Read the model definition and answer for the solid it produces. Units are mm, in the model's axes. Face numbers are marked on the shaded views. A direction names the side the tool comes from. Coordinates: 2 decimals unless noted, no trailing zeros. Order: outer loops, then holes, each group sorted by start corner. A loop starts at its lowest first (then second) coordinate and runs counter-clockwise, first axis right, second up. Notation, with made-up numbers: (42.25, -16) - (76.25, -16) arc R9 cw to (76.25, -11) - close; hole circle Ø4 at (24.5, -40). An arc over 180 degrees is marked (long way). Write item = value, one per line.
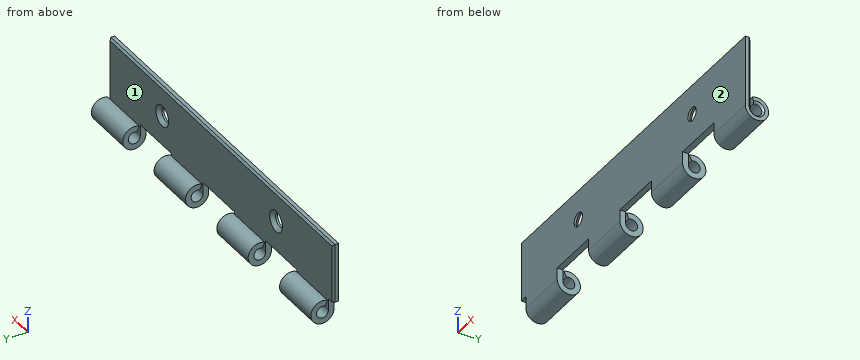
from build123d import *

# Parameters (mm, degrees)
SKETCH1_W          = 100
SKETCH1_H          = 22.1615
BASE_FLANGE1_DEPTH = 1.524
HEM1_START         = -50
HEM1_DEPTH         = 100
HEM1_2_DEPTH       = 100
CUT_EXTRUDE1_START = -52.42823759
SKETCH8_W          = 14
SKETCH8_H          = 6.223
CUT_EXTRUDE1_DEPTH = 94.856475179
LPATTERN1_COUNT    = 11
LPATTERN1_PITCH    = 28
CHAMFER1_SIZE      = 0.5
SKETCH9_R          = 1.8288
CUT_EXTRUDE2_DEPTH = 10
LPATTERN2_COUNT    = 6
LPATTERN2_PITCH    = 50.8
CHAMFER2_SIZE      = 1


# Read off the part's stored shape, not the designer's step: Hem1
# Sheet-metal steps are written as plain solids
with BuildPart() as part:
    # Sketch1 → Base-Flange1 (new body)
    with BuildSketch(Plane(origin=(0, 0, 0), x_dir=(1, 0, 0), z_dir=(0, 1, 0))):
        Rectangle(SKETCH1_W, SKETCH1_H)
    extrude(amount=-BASE_FLANGE1_DEPTH)

    # Hem1 outline → Hem1 (cut)
    with BuildSketch(Plane.YZ.offset(HEM1_START)):
        with BuildLine():
            Line((0, -11.08075), (0, -10.645306054))
            ThreePointArc((0, -10.645306054), (-1.116287945, -9.509043168), (-1.524, -7.96925))
            Line((-1.524, -7.96925), (-1.524, -11.08075))
            Line((-1.524, -11.08075), (0, -11.08075))
        make_face()
    extrude(amount=HEM1_DEPTH, mode=Mode.SUBTRACT)

    # Hem1 2 outline → Hem1 2 (add)
    with BuildSketch(Plane.YZ.offset(HEM1_START)):
        with BuildLine():
            Line((0.272523279, -5.149273321), (0.916593509, -6.530486388))
            ThreePointArc((0.916593509, -6.530486388), (2.92638392, -8.822213128), (0, -7.96925))
            Line((0, -7.96925), (0, -10.645306054))
            ThreePointArc((0, -10.645306054), (4.69518189, -8.123345818), (0.272523279, -5.149273321))
        make_face()
    extrude(amount=HEM1_2_DEPTH)

    # Sketch8 → Cut-Extrude1 (cut)
    with BuildSketch(Plane(origin=(0, 0, 0), x_dir=(1, 0, 0), z_dir=(0, 1, 0)).offset(CUT_EXTRUDE1_START)):
        with Locations((29, 7.96925)):
            Rectangle(SKETCH8_W, SKETCH8_H)
    cut_extrude1 = extrude(amount=CUT_EXTRUDE1_DEPTH, mode=Mode.SUBTRACT)

    # LPattern1: Cut-Extrude1 ×11
    with Locations(*[(-i * LPATTERN1_PITCH, 0, 0) for i in range(1, LPATTERN1_COUNT)]):
        add(cut_extrude1, mode=Mode.SUBTRACT)

    # Chamfer1
    chamfer1_edges = [part.edges().sort_by_distance(p)[0] for p in [
        (-50, 0, 3.1115),
        (50, 2.92638392, -8.822213128),
        (0, 0, 11.08075),
        (50, 0, 1.55575),
    ]]
    chamfer(chamfer1_edges, length=CHAMFER1_SIZE)

    # Sketch9 → Cut-Extrude2 (cut)
    with BuildSketch(Plane(origin=(0, 0, 0), x_dir=(1, 0, 0), z_dir=(0, 1, 0))):
        with Locations(Location((-24.6, -3.14325, 0), (0, 0, 270))):
            Circle(SKETCH9_R)
    cut_extrude2 = extrude(amount=-CUT_EXTRUDE2_DEPTH, mode=Mode.SUBTRACT)

    # LPattern2: Cut-Extrude2 ×6
    with Locations(*[(i * LPATTERN2_PITCH, 0, 0) for i in range(1, LPATTERN2_COUNT)]):
        add(cut_extrude2, mode=Mode.SUBTRACT)

    # Chamfer2
    chamfer2_edges = [part.edges().sort_by_distance(p)[0] for p in [
        (-24.6, 0, 1.31445),
        (26.2, 0, 1.31445),
    ]]
    chamfer(chamfer2_edges, length=CHAMFER2_SIZE)


solid = part.part
1) For the marked faces 1 and 2, determine the directions among +Z, -Z, +X, -X, +Y, -Y from which every point of the face is accessible in a straight line to the end or side of a thin tool.
Returned:
face_1 = +Z, +X, -X
face_2 = +Z, -Z, +X, -X, -Y
2) Flat-ended cylindrical pins translate along their axes: pin 1 Ø3 at (y, z) = (3, -8.5) entering from -X; pin 2 Ø3 at (y, z) = (1.59, -7.97) entering from -X; pin 3 Ø0.5 at (x, y) = (-24.5, -0.5) entering from -Z; pin 4 Ø1 at (x, z) = (22.5, 6) entering from +Y. Find the tip coordinate at first contact, or state that the pin passes through.
Returned:
pin_1 = -48
pin_2 = through
pin_3 = -4.86
pin_4 = 0
3) The part is cut by section C-C (z = -3). Determine the outline of the cut face in (x, y).
Returned:
outline = (-50, -1.52) - (50, -1.52) - (50, -0.5) - (49.5, 0) - (-49.5, 0) - (-50, -0.5) - close
4) The part is cut by section A-A (x = 26.2). Determine the outline of the cut face in (y, z), and give its area (3 significant figures).
Returned:
outline = (-1.52, -4.86) - (0, -4.86) - (0, 0.31) - (-1, 1.31) - (-1.52, 1.31) - close; (-1.52, 4.97) - (-1, 4.97) - (0, 5.97) - (0, 10.58) - (-0.5, 11.08) - (-1.52, 11.08) - close
area = 17.6 mm^2
5) The part is cut by section B-B (x = -35.5). Determine the outline of the cut face in (y, z) (1 decimal), and give its area (3 significant figures).
Returned:
outline = (-1.5, -8) arc R3.1 ccw (long way) to (0.3, -5.1) - (0.9, -6.5) arc R1.6 cw (long way) to (0, -8) - (0, 10.6) - (-0.5, 11.1) - (-1.5, 11.1) - close
area = 47.3 mm^2
6) Straight lines are drawn through the part: line 1 along X through (y, z) = (3.75, -8.5); line 2 along Y through (x, z) = (-10, -8); line 3 along Y through (x, z) = (-18.5, 0.5). For each, find the intervals that lie inside material, in ascending order. Write a range as from..to.
Returned:
line_1 = -48..-34, -20..-6, 8..22, 36..50
line_2 = -1.52..0, 3.17..4.7
line_3 = -1.52..0
